Here's how the part is built. I have some questions about the finished solid (model axes, mm). Round coordinates to 2 decimals unless told otherwise and drop trailing zeros. Write each loop counter-clockwise with the first axis right and the second up, starting at its lowest first coordinate (ties: lowest second). Pieces come first, ordered by that corner, then holes. Notation, with made-up numbers: (46, 2) -> (90, 2) arc R25 cw to (90, 27) -> close; hole circle Ø3 at (-26.5, 24). An arc over 180 degrees is marked (long way). Put each result on its own line as item: value. Start each with the question number.
1) If I drill on line 1 along Y through (x, z) = (126.5, 1.8); line 2 along Y through (x, z) = (149.5, 2.65); line 3 along X through (y, z) = (-4.75, 2.9), over which ranges is the centre line in solid material (lowest first)? Write a range as [from, to].
2) I want a section at A-A, the plane y = -1.75. List the corners of the cut face in (x, z) for me (3 decimals).
3) We'd pull the mould along Y, two halves only. Please class faces 1 (the flat face through (118.95, 0.69, 1.61)), 2 (the flat face through (162.765, -4.836, 1.61)), 3 (the flat face through (146, 1, 3.175)): released by +Y, released by -Y, zero draft, split by the parting line, or undercut.
from build123d import *

# Parameters (mm, degrees)
BOSS_EXTRUDE1_DEPTH = 3.175
CUT_EXTRUDE1_DEPTH  = 5.08


with BuildPart() as part:
    # Sketch2 → Boss-Extrude1 (new body)
    with BuildSketch(Plane.XY):
        with BuildLine():
            add(Edge.make_bspline(
                [(213.36, 0), (213.257272793, 0.119144956), (212.930217359, 0.49847003), (211.784320833, 0.388103102), (210.220456583, 0.752231195), (207.922221089, 1.002358459), (205.040435451, 1.416814194), (201.53687476, 1.872417288), (197.453852985, 2.405608245), (192.809425036, 2.993232985), (187.634552437, 3.632300405), (181.96038472, 4.311820743), (175.822180186, 5.024095776), (169.257621951, 5.759205624), (162.307240439, 6.508241756), (155.013925984, 7.261881453), (147.42262952, 8.010402764), (139.580173762, 8.743297071), (131.534856191, 9.450943444), (123.336366748, 10.121511173), (115.035081585, 10.744066661), (106.682256297, 11.307051658), (98.329355975, 11.798694638), (90.027802971, 12.206574858), (81.828867412, 12.519815813), (73.782861936, 12.728198408), (65.939509207, 12.821544448), (58.347003411, 12.792445951), (51.052154229, 12.635282307), (44.099865123, 12.34606959), (37.532927606, 11.924051264), (31.391706263, 11.370497155), (25.713767757, 10.689730544), (20.533764615, 9.887543747), (15.882945038, 8.97231492), (11.789015751, 7.954392799), (8.273858988, 6.843703394), (5.359469774, 5.650591236), (3.043164975, 4.383128287), (1.36213983, 3.038812968), (0.222897845, 1.585123236), (0.070856618, 0.503892135), (0, 0)],
                knots=[0, 0, 0, 0, 0.002091853, 0.006659889, 0.014240034, 0.024784942, 0.038226646, 0.054481348, 0.073444809, 0.094998776, 0.11900639, 0.145318898, 0.173770288, 0.204183654, 0.236370679, 0.270129473, 0.305250351, 0.341516861, 0.378701149, 0.416575318, 0.454902219, 0.493447217, 0.531971459, 0.57023708, 0.608012632, 0.645066312, 0.681178002, 0.716129843, 0.74971807, 0.781748295, 0.812036536, 0.840415327, 0.866732056, 0.890849065, 0.912651845, 0.932046273, 0.94897292, 0.963413199, 0.975421325, 0.985175212, 0.993091122, 1, 1, 1, 1], degree=3))
            add(Edge.make_bspline(
                [(213.36, 0), (213.257272793, -0.119144956), (212.930217359, -0.49847003), (211.784320833, -0.388103102), (210.220456583, -0.752231195), (207.922221089, -1.002358459), (205.040435451, -1.416814194), (201.53687476, -1.872417288), (197.453852985, -2.405608245), (192.809425036, -2.993232985), (187.634552437, -3.632300405), (181.96038472, -4.311820743), (175.822180186, -5.024095776), (169.257621951, -5.759205624), (162.307240439, -6.508241756), (155.013925984, -7.261881453), (147.42262952, -8.010402764), (139.580173762, -8.743297071), (131.534856191, -9.450943444), (123.336366748, -10.121511173), (115.035081585, -10.744066661), (106.682256297, -11.307051658), (98.329355975, -11.798694638), (90.027802971, -12.206574858), (81.828867412, -12.519815813), (73.782861936, -12.728198408), (65.939509207, -12.821544448), (58.347003411, -12.792445951), (51.052154229, -12.635282307), (44.099865123, -12.34606959), (37.532927606, -11.924051264), (31.391706263, -11.370497155), (25.713767757, -10.689730544), (20.533764615, -9.887543747), (15.882945038, -8.97231492), (11.789015751, -7.954392799), (8.273858988, -6.843703394), (5.359469774, -5.650591236), (3.043164975, -4.383128287), (1.36213983, -3.038812968), (0.222897845, -1.585123236), (0.070856618, -0.503892135), (0, 0)],
                knots=[0, 0, 0, 0, 0.002091853, 0.006659889, 0.014240034, 0.024784942, 0.038226646, 0.054481348, 0.073444809, 0.094998776, 0.11900639, 0.145318898, 0.173770288, 0.204183654, 0.236370679, 0.270129473, 0.305250351, 0.341516861, 0.378701149, 0.416575318, 0.454902219, 0.493447217, 0.531971459, 0.57023708, 0.608012632, 0.645066312, 0.681178002, 0.716129843, 0.74971807, 0.781748295, 0.812036536, 0.840415327, 0.866732056, 0.890849065, 0.912651845, 0.932046273, 0.94897292, 0.963413199, 0.975421325, 0.985175212, 0.993091122, 1, 1, 1, 1], degree=3))
        make_face()
    extrude(amount=BOSS_EXTRUDE1_DEPTH)

    # Sketch3 → Cut-Extrude1 (cut)
    with BuildSketch(Plane.XY.offset(3.175)):
        Polygon((111.76, 10.961711107), (126.348178921, -9.872367542), (126.348178921, -50.8), (0, -50.8), (0, 0), (0, 50.8), (111.76, 50.8), align=None)
        Polygon((163.371025422, -9.582434223), (213.762062152, -3.149439796), (212.957937848, 3.149439796), (162.566901119, -3.283554632), align=None)
    extrude(amount=-CUT_EXTRUDE1_DEPTH, mode=Mode.SUBTRACT)


solid = part.part
Findings:
1. line 1: y = [-9.86, 9.86]
1. line 2: y = [-7.8, 7.8]
1. line 3: x = [122.76, 162.75]
2. outline: (120.661, 0) -> (174.58, 0) -> (174.58, 3.175) -> (120.661, 3.175) -> close
3. face 1: released by -Y
3. face 2: undercut
3. face 3: zero draft
